Read the model definition and answer for the solid it produces. Units are mm, in the model's axes. Face numbers are marked on the shaded views. A direction names the side the tool comes from. Round coordinates to 2 decimals unless told otherwise and drop trailing zeros. Write each loop counter-clockwise with the first axis right and the second up, starting at its lowest first coordinate (ties: lowest second). Pieces come first, ordered by that corner, then holes. Notation, with made-up numbers: (-6.75, 77) - (34.25, 77) arc R25 cw to (34.25, 101) - close; hole circle Ø9 at (84, 80). An arc over 180 degrees is marked (long way). One line per item, written item: value. Start each with the question number.
(1) Find the intervals of material crossed by L1, parallel to Y at x = 24.5, z = -31; L2, parallel to X at y = 8, z = -35.5; L3, parallel to Z at x = 2.5, y = 9.5, in increasing order.
(2) A cutting plane is placed at D-D, the plane x = 7. Determine the outline of the cut face in (y, z).
(3) For the marked faces 1, 2 and 3, determine the directions among +Z, -Z, +X, -X, +Y, -Y from which every point of the face is accessible in a straight line to the end or side of a thin tool.
(4) The mould has two halves that part along Y. Classify the marked faces 4, 5 and 6: +Y half, -Y half, draft (parallel to the pull), parting line (faces both ways), or undercut.
(5) A cutting plane is placed at C-C, the plane y = 24.5. Determine the outline of the cut face in (x, z).
(6) A cutting plane is placed at A-A, the plane z = -27. Determine the outline of the cut face in (x, y).
(7) Flat-ended cylindrical pins translate along their axes: pin 1 Ø10 at (x, y) = (34.5, 13) entering from +Z; pin 2 Ø2.5 at (x, z) = (39, -20) entering from +Y; pin 3 Ø10.5 at (x, y) = (11, 16) entering from -Z. Find the tip coordinate at first contact, or state that the pin passes through.
(8) A cutting plane is placed at B-B, the plane x = 23. Determine the outline of the cut face in (y, z), plus the area to 3 significant figures.
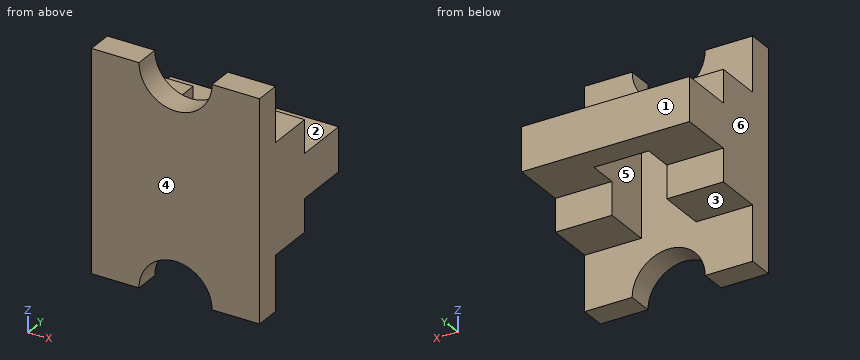
from build123d import *

# Parameters (mm, degrees)
SKETCH1_W               = 12
SKETCH1_H               = 7
BOSS_EXTRUDE1_DEPTH     = 46
CUT_EXTRUDE2_DEPTH      = 46
CUT_EXTRUDE2_DEPTH_BACK = 46
SKETCH6_W               = 15
SKETCH6_H               = 21
CUT_EXTRUDE3_DEPTH      = 60


with BuildPart() as part:
    # Sketch1 → Boss-Extrude1 (new body)
    with BuildSketch(Plane(origin=(0, 0, 0), x_dir=(0, 0, -1), z_dir=(1, 0, 0))):
        with Locations((30, 31.5)):
            Rectangle(SKETCH1_W, SKETCH1_H)
        Polygon((0, 7), (0, 0), (60, 0), (60, 7), (45, 7), (45, 20), (36, 20), (36, 28), (24, 28), (24, 20), (15, 20), (15, 7), align=None)
    extrude(amount=BOSS_EXTRUDE1_DEPTH)

    # Sketch2 → Cut-Extrude2 (cut, two sides: drawn at the far end of the back side and taken through both)
    with BuildSketch(Plane(origin=(0, 0, 0), x_dir=(1, 0, 0), z_dir=(0, 1, 0)).offset(-CUT_EXTRUDE2_DEPTH_BACK)):
        with BuildLine():
            ThreePointArc((33, 0), (23, 10), (13, 0))
            Line((13, 0), (33, 0))
        make_face()
        with BuildLine():
            Line((33, 0), (13, 0))
            ThreePointArc((13, 0), (23, -10), (33, 0))
        make_face()
        with BuildLine():
            ThreePointArc((33, 60), (23, 70), (13, 60))
            Line((13, 60), (33, 60))
        make_face()
        with BuildLine():
            Line((33, 60), (13, 60))
            ThreePointArc((13, 60), (23, 50), (33, 60))
        make_face()
    extrude(amount=CUT_EXTRUDE2_DEPTH + CUT_EXTRUDE2_DEPTH_BACK, mode=Mode.SUBTRACT)

    # Sketch6 → Cut-Extrude3 (cut)
    with BuildSketch(Plane.XY):
        with Locations((23, 17.5)):
            Rectangle(SKETCH6_W, SKETCH6_H)
    extrude(amount=-CUT_EXTRUDE3_DEPTH, mode=Mode.SUBTRACT)


solid = part.part
Here are the results:
1. L1: 0 to 7, 28 to 35
1. L2: 0 to 15.5, 30.5 to 46
1. L3: -45 to -15
2. outline: (0, -60) - (7, -60) - (7, -45) - (20, -45) - (20, -36) - (35, -36) - (35, -24) - (20, -24) - (20, -15) - (7, -15) - (7, 0) - (0, 0) - close
3. face 1: +Z, -Z, +X, -X, +Y
3. face 2: +Z, +X, -X, +Y
3. face 3: -Z, +X, -X, +Y
4. face 4: -Y half
4. face 5: undercut
4. face 6: draft
5. outline: (0, -36) - (15.5, -36) - (15.5, -24) - (0, -24) - close; (30.5, -36) - (46, -36) - (46, -24) - (30.5, -24) - close
6. outline: (0, 0) - (46, 0) - (46, 35) - (0, 35) - close; hole (15.5, 7) - (30.5, 7) - (30.5, 28) - (15.5, 28) - close
7. pin 1: z = -15
7. pin 2: y = 20
7. pin 3: z = -45
8. outline: (0, -50) - (7, -50) - (7, -10) - (0, -10) - close; (28, -36) - (35, -36) - (35, -24) - (28, -24) - close
8. area: 364 mm²
